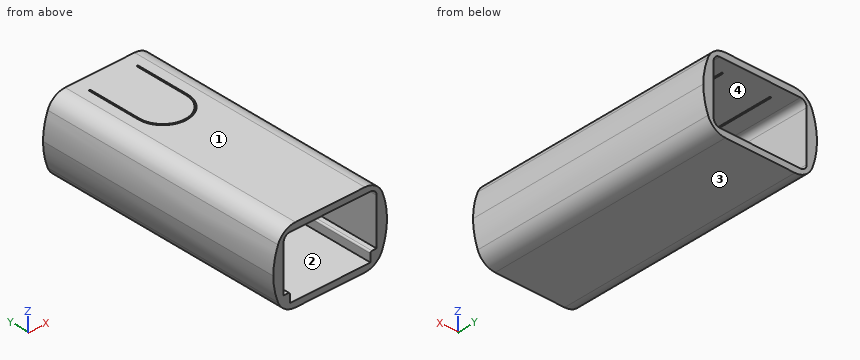
```python
from build123d import *

# Parameters (mm, degrees)
BOSS_EXTRUDE4_DEPTH = 80
BOSS_EXTRUDE5_DEPTH = 57
CUT_EXTRUDE1_DEPTH  = 2
CHAMFER1_SIZE       = 2.83564091
CHAMFER1_SIZE_2     = 0.5


with BuildPart() as part:
    # Sketch8 → Boss-Extrude4 (new body)
    with BuildSketch(Plane(origin=(0, 58, 0), x_dir=(1, 0, 0), z_dir=(0, 1, 0))):
        with BuildLine():
            Line((-11.194828593, 12.000000011), (11.194828559, 12.000000011))
            ThreePointArc((11.194828559, 12.000000011), (14.611088941, 10.932460351), (16.811684841, 8.109721678))
            add(Edge.make_bspline(
                [(18.334712564, 1.1e-08), (18.327162677, 2.726130673), (17.819510816, 5.426517656), (16.811684841, 8.109721678)],
                knots=[0.502499344, 0.502499344, 0.502499344, 0.502499344, 0.837905074, 0.837905074, 0.837905074, 0.837905074], degree=3))
            add(Edge.make_bspline(
                [(18.334712564, 1.1e-08), (18.327162677, -2.72613065), (17.819510816, -5.426517634), (16.811684841, -8.109721656)],
                knots=[0.502499344, 0.502499344, 0.502499344, 0.502499344, 0.837905074, 0.837905074, 0.837905074, 0.837905074], degree=3))
            ThreePointArc((16.811684841, -8.109721656), (14.611088941, -10.932460328), (11.194828559, -11.999999989))
            Line((11.194828559, -11.999999989), (-11.194828593, -11.999999989))
            ThreePointArc((-11.194828593, -11.999999989), (-14.611088975, -10.932460328), (-16.811684874, -8.109721656))
            add(Edge.make_bspline(
                [(-18.334712598, 1.1e-08), (-18.327162711, -2.72613065), (-17.81951085, -5.426517634), (-16.811684874, -8.109721656)],
                knots=[0.502499344, 0.502499344, 0.502499344, 0.502499344, 0.837905074, 0.837905074, 0.837905074, 0.837905074], degree=3))
            add(Edge.make_bspline(
                [(-18.334712598, 1.1e-08), (-18.327162711, 2.726130673), (-17.81951085, 5.426517656), (-16.811684874, 8.109721678)],
                knots=[0.502499344, 0.502499344, 0.502499344, 0.502499344, 0.837905074, 0.837905074, 0.837905074, 0.837905074], degree=3))
            ThreePointArc((-16.811684874, 8.109721678), (-14.611088975, 10.932460351), (-11.194828593, 12.000000011))
        make_face()
        with BuildLine():
            Line((-15.000000017, -7.999999989), (-15.000000017, 8.000000011))
            ThreePointArc((-15.000000017, 8.000000011), (-14.414213579, 9.414213574), (-13.000000017, 10.000000011))
            Line((-13.000000017, 10.000000011), (12.999999983, 10.000000011))
            ThreePointArc((12.999999983, 10.000000011), (14.414213546, 9.414213574), (14.999999983, 8.000000011))
            Line((14.999999983, 8.000000011), (14.999999983, -7.999999989))
            ThreePointArc((14.999999983, -7.999999989), (14.414213546, -9.414213551), (12.999999983, -9.999999989))
            Line((12.999999983, -9.999999989), (-13.000000017, -9.999999989))
            ThreePointArc((-13.000000017, -9.999999989), (-14.414213579, -9.414213551), (-15.000000017, -7.999999989))
        make_face(mode=Mode.SUBTRACT)
    extrude(amount=BOSS_EXTRUDE4_DEPTH)

    # Sketch11 → Boss-Extrude5 (add)
    with BuildSketch(Plane(origin=(0, 58, 0), x_dir=(1, 0, 0), z_dir=(0, 1, 0))):
        with BuildLine():
            Line((13, 10.000000011), (15, 10.000000011))
            Line((15, 10.000000011), (15, 6.937911183))
            Line((15, 6.937911183), (13.5, 6.937911183))
            ThreePointArc((13.5, 6.937911183), (13.146446609, 7.084357793), (13, 7.437911183))
            Line((13, 7.437911183), (13, 10.000000011))
        make_face()
        with BuildLine():
            Line((-13, 7.437911183), (-13, 10.000000011))
            Line((-13, 10.000000011), (-15, 10.000000011))
            Line((-15, 10.000000011), (-15, 6.937911183))
            Line((-15, 6.937911183), (-13.5, 6.937911183))
            ThreePointArc((-13.5, 6.937911183), (-13.146446609, 7.084357793), (-13, 7.437911183))
        make_face()
    extrude(amount=BOSS_EXTRUDE5_DEPTH)

    # Sketch12 → Cut-Extrude1 (cut)
    with BuildSketch(Plane.XY.offset(11.999999989)):
        with BuildLine():
            Line((7.5, 133.134156445), (7.5, 116.134156445))
            ThreePointArc((7.5, 116.134156445), (0, 108.634156445), (-7.5, 116.134156445))
            Line((-7.5, 116.134156445), (-7.5, 133.134156445))
            ThreePointArc((-7.5, 133.134156445), (-7.75, 133.384156445), (-8, 133.134156445))
            Line((-8, 133.134156445), (-8, 116.134156445))
            ThreePointArc((-8, 116.134156445), (0, 108.134156445), (8, 116.134156445))
            Line((8, 116.134156445), (8, 133.134156445))
            ThreePointArc((8, 133.134156445), (7.75, 133.384156445), (7.5, 133.134156445))
        make_face()
    extrude(amount=-CUT_EXTRUDE1_DEPTH, mode=Mode.SUBTRACT)

    # Chamfer1
    # the kernel refuses this chamfer: 2.83564091, 0.5 mm, written as the material it takes off along each edge
    with BuildSketch(Plane(origin=(13, 115, -7.437911183), x_dir=(0, -1, 0), z_dir=(0, 0, -1))) as chamfer1_piece_1_section:
        Polygon((CHAMFER1_SIZE, 0), (0, -CHAMFER1_SIZE_2), (0, 0), align=None)
    chamfer1_piece_1 = extrude(amount=9.930611745, mode=Mode.PRIVATE)
    chamfer1_piece_1 = chamfer1_piece_1 & Plane(origin=(12.999999983, 115, -8.000000011), x_dir=(0, 0, -1), z_dir=(0, -1, 0)) * Cylinder(2, 32, mode=Mode.PRIVATE)
    add(chamfer1_piece_1, mode=Mode.SUBTRACT)
    with BuildSketch(Plane(origin=(13.5, 115, -7.437911183), x_dir=(0, 0, 1), z_dir=(1, 0, 0))) as chamfer1_piece_2:
        Polygon((0.5, CHAMFER1_SIZE), (0.5 - CHAMFER1_SIZE_2, 0), (0.5, 0), align=None)
    revolve(axis=Axis((13.5, 115, -7.437911183), (0, -1, 0)), revolution_arc=90, mode=Mode.SUBTRACT)
    with BuildSketch(Plane(origin=(15, 115, -6.937911183), x_dir=(0, -1, 0), z_dir=(-1, 0, 0))) as chamfer1_piece_3:
        Polygon((CHAMFER1_SIZE, 0), (0, -CHAMFER1_SIZE_2), (0, 0), align=None)
    extrude(amount=1.5, mode=Mode.SUBTRACT)
    with BuildSketch(Plane(origin=(-13, 115, -7.437911183), x_dir=(0, -1, 0), z_dir=(0, 0, -1))) as chamfer1_piece_4_section:
        Polygon((CHAMFER1_SIZE, 0), (0, CHAMFER1_SIZE_2), (0, 0), align=None)
    chamfer1_piece_4 = extrude(amount=9.930611745, mode=Mode.PRIVATE)
    chamfer1_piece_4 = chamfer1_piece_4 & Plane(origin=(-13.000000017, 115, -8.000000011), x_dir=(-1, 0, 0), z_dir=(0, -1, 0)) * Cylinder(2, 32, mode=Mode.PRIVATE)
    add(chamfer1_piece_4, mode=Mode.SUBTRACT)
    with BuildSketch(Plane(origin=(-15, 115, -6.937911183), x_dir=(0, -1, 0), z_dir=(1, 0, 0))) as chamfer1_piece_5:
        Polygon((CHAMFER1_SIZE, 0), (0, CHAMFER1_SIZE_2), (0, 0), align=None)
    extrude(amount=1.5, mode=Mode.SUBTRACT)
    with BuildSketch(Plane(origin=(-13.5, 115, -7.437911183), x_dir=(0, 0, 1), z_dir=(-1, 0, 0))) as chamfer1_piece_6:
        Polygon((0.5, -CHAMFER1_SIZE), (0.5 - CHAMFER1_SIZE_2, 0), (0.5, 0), align=None)
    revolve(axis=Axis((-13.5, 115, -7.437911183), (0, 1, 0)), revolution_arc=90, mode=Mode.SUBTRACT)


solid = part.part
```
Here's how the part is built. I have some questions about the finished solid (model axes, mm). Face numbers are marked on the shaded views. Give positions to 0.01 mm unless a question says otherwise; leave off trailing zeros. Order: outer loops, then holes, each group sorted by start corner. A loop starts at its lowest first (then second) coordinate and runs counter-clockwise, first axis right, second up. Notation, with made-up numbers: (55.5, 31.25) -> (80.5, 31.25) arc R19 cw to (80.5, 53.25) -> close; hole circle Ø4 at (26, -16). An arc over 180 degrees is marked (long way). Use CSV: the item, a comma, the result in double quotes. Start each with the question number.
Item 1: If I drill on probe 1 along Z at (x, y) = (4, 103.5); probe 2 along X at (y, z) = (87, 4.75); probe 3 along X at (y, z) = (78, -3.75), over which ranges is the centre line in solid material (lowest first)? Write a range as [from, to].
Item 2: I'm going to push flat-ended pins straight in: P1, Ø1.7, axis at x = -14, z = -9.5, coming from the +Y side; P2, Ø1.3, axis at y = 92, z = -9, coming from the +X side; P3, Ø1.6, axis at x = -14, y = 95.5, coming from the +Z side (3 decimals); P4, Ø1, axis at y = 127, z = 11.5, coming from the -X side. Where does each tip first touch, or does it pass through?
Item 3: Thinking about a two-plate mould opening in Z: for the marked faces 1, 2, 3 and 4, which applies, pulls with the +Z half, pulls with the -Z half, needs draft (parallel to the pull), parting line crosses it, or undercut?
Item 4: Suppose I cut it at A-A (x = 0). List the corners of the cut face in (y, z) for me.
Answer block:
1,probe 1,"z = [-12, -10], [10, 12]"
1,probe 2,"x = [-17.81, -15], [15, 17.81]"
1,probe 3,"x = [-18.01, -15], [15, 18.01]"
2,P1,"stops at y = 138"
2,P2,"stops at x = 16.72"
2,P3,"stops at z = 11.655"
2,P4,"stops at x = -14.51"
3,face 1,"pulls with the +Z half"
3,face 2,"undercut"
3,face 3,"pulls with the -Z half"
3,face 4,"undercut"
4,outline,"(58, -12) -> (138, -12) -> (138, -10) -> (58, -10) -> close; (58, 10) -> (108.13, 10) -> (108.13, 12) -> (58, 12) -> close; (108.63, 10) -> (138, 10) -> (138, 12) -> (108.63, 12) -> close"
